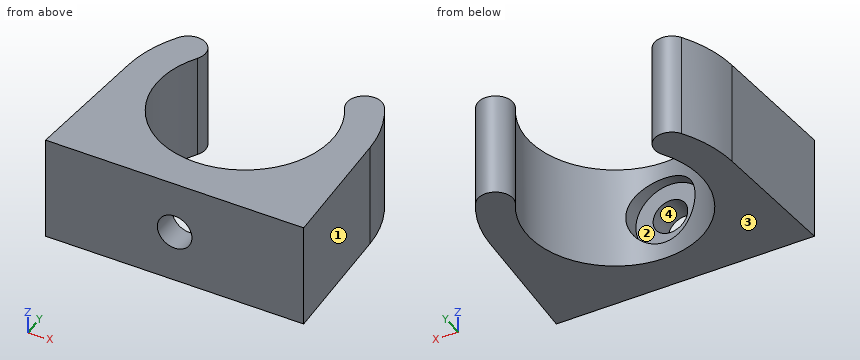
```python
from build123d import *

# Parameters (mm, degrees)
F1_DEPTH       = 15
F4_D           = 5
F4_START       = 12.5000001
F4_CBORE_D     = 10
F4_CBORE_DEPTH = 1.5


# Not quite as in the source:
# - a feature of the source that left no trace in its solid (it failed there, or was rolled back) is left out


with BuildPart() as f1:
    # F0 (on Top) → F1 (new body)
    with BuildSketch(Plane.XY):
        with BuildLine():
            ThreePointArc((10.6047668571, 35.4310178135), (0.0084014235, 16.3137009448), (-10.6136524588, 35.4167566161))
            ThreePointArc((-10.6136524588, 35.4167566161), (-11.4157712516, 38.8600988068), (-14.8591134423, 38.057980014))
            ThreePointArc((-14.8591134423, 38.057980014), (-16.6714054435, 34.1348108377), (-17.4670460885, 29.8871509353))
            Line((-17.4670460885, 29.8871509353), (-18.6252595091, 11.0408943146))
            Line((-18.6252595091, 11.0408943146), (18.6252595091, 11.0408943146))
            Line((18.6252595091, 11.0408943146), (17.4670460885, 29.8871509353))
            ThreePointArc((17.4670460885, 29.8871509353), (16.6678252842, 34.1460147189), (14.8466735999, 38.0779456904))
            ThreePointArc((14.8466735999, 38.0779456904), (11.4022562901, 38.8754351234), (10.6047668571, 35.4310178135))
        make_face()
    extrude(amount=F1_DEPTH)

    # F4 (through all)
    # its depths count from where the whole tool has entered the part; down to there all is cleared
    with Locations(Plane(origin=(0, 28.8136981214, 0), x_dir=(-1, 0, 0), z_dir=(0, 1, 0)).offset(-F4_START)):
        with Locations((0, 7.5)):
            CounterBoreHole(F4_D / 2, F4_CBORE_D / 2, F4_CBORE_DEPTH)


solid = f1.part
```
The model under review builds one solid part; all positions refer to its coordinate system, in mm. Face numbers are marked on the shaded views. Round coordinates to 2 decimals unless told otherwise and drop trailing zeros. Write each loop counter-clockwise with the first axis right and the second up, starting at its lowest first coordinate (ties: lowest second). Pieces come first, ordered by that corner, then holes.
(1) We need section B-B on z = 7.5. Give the boundary of the cut face in (x, y), and give its area (3 significant figures).
(2) We need section C-C on y = 20.5. Give the boundary of the cut face in (x, z), and give its area (3 significant figures).
(3) Insertion check: pin 1 (1.5 mm diameter, centred on x = -9, z = 2.5, fed in from +Y); pin 2 (2 mm diameter, centred on y = 33.5, z = 2.5, fed in from +X). Each pin has a flat end and moves straight along its axis. Give the tip position at first contact, or say it passes through.
(4) We need section D-D on z = 11. Give the boundary of the cut face in (x, y).
(5) We need section A-A on x = 0. Give the boundary of the cut face in (y, z), and give its area (3 significant figures).
(6) Wall thickness on L1, parallel to Z at x = 0, y = 12.3; L2, parallel to Z at x = 0, y = 15.55; L3, parallel to Y at x = 0, z = 4: over which ranges is each line inside the solid? List them lowest first.
(7) Mouldability with a two-part tool opening along Z and no side actions: class the marked faces 1, 2, 3 and 4 as +Z half, -Z half, draft (parallel to the pull), parting line (faces both ways), or undercut.
Findings below:
1. outline: (-18.63, 11.04) - (-2.5, 11.04) - (-2.5, 14.81) - (-5, 14.81) - (-5, 17.36) arc R12.5 cw to (-10.61, 35.42) arc R2.5 ccw to (-14.86, 38.06) arc R17.5 ccw to (-17.47, 29.89) - close; (2.5, 11.04) - (18.63, 11.04) - (17.47, 29.89) arc R17.5 ccw to (14.85, 38.08) arc R2.5 ccw to (10.6, 35.43) arc R12.5 cw to (5, 17.36) - (5, 14.81) - (2.5, 14.81) - close
1. area: 463 mm2
2. outline: (-18.04, 0) - (-9.33, 0) - (-9.33, 15) - (-18.04, 15) - close; (9.33, 0) - (18.04, 0) - (18.04, 15) - (9.33, 15) - close
2. area: 261 mm2
3. pin 1: stops at y = 20.99
3. pin 2: stops at x = 17.11
4. outline: (-18.63, 11.04) - (18.63, 11.04) - (17.47, 29.89) arc R17.5 ccw to (14.85, 38.08) arc R2.5 ccw to (10.6, 35.43) arc R12.5 cw to (3.57, 16.83) - (3.57, 14.81) - (-3.57, 14.81) - (-3.57, 16.83) arc R12.5 cw to (-10.61, 35.42) arc R2.5 ccw to (-14.86, 38.06) arc R17.5 ccw to (-17.47, 29.89) - close
5. outline: (11.04, 0) - (16.31, 0) - (16.31, 2.5) - (14.81, 2.5) - (14.81, 5) - (11.04, 5) - close; (11.04, 10) - (14.81, 10) - (14.81, 12.5) - (16.31, 12.5) - (16.31, 15) - (11.04, 15) - close
5. area: 45.2 mm2
6. L1: z = 0 to 5, 10 to 15
6. L2: z = 0 to 2.5, 12.5 to 15
6. L3: y = 11.04 to 14.81
7. face 1: draft
7. face 2: undercut
7. face 3: -Z half
7. face 4: undercut
